```python
from build123d import *

# Parameters (mm, degrees)
MODEL_R             = 1.62599878
MODEL_W             = 8.89
MODEL_H             = 6.096
EXTRUDE_1_DEPTH     = 1
EXTRUDE_2_DEPTH     = 3
SKETCH_1_W          = 8.89
SKETCH_1_H          = 1
EXTRUDE_3_DEPTH     = 0.5
SKETCH_2_W          = 1
SKETCH_2_H          = 5.207
EXTRUDE_4_DEPTH     = 0.5
SKETCH_3_W          = 1
SKETCH_3_H          = 5.207
EXTRUDE_5_DEPTH     = 0.5
SKETCH_4_W          = 7.636
SKETCH_4_H          = 1
CUT_EXTRUDE_1_DEPTH = 0.5


with BuildPart() as part:
    # Model → Extrude 1 (new body)
    with BuildSketch(Plane.XY):
        with BuildLine():
            Line((122.15333456, 67.05953568), (122.15333456, 103.29453306))
            ThreePointArc((122.15333456, 103.29453306), (119.410664993, 110.045001733), (112.66019632, 112.7876713))
            Line((112.66019632, 112.7876713), (83.7431777, 112.7876713))
            ThreePointArc((83.7431777, 112.7876713), (77.016609687, 110.107501601), (74.21120032, 103.43219598))
            Line((74.21120032, 103.43219598), (74.21120032, 67.1865433))
            ThreePointArc((74.21120032, 67.1865433), (76.909728462, 60.481379821), (83.57819454, 57.69339998))
            Line((83.57819454, 57.69339998), (112.78719886, 57.69339998))
            ThreePointArc((112.78719886, 57.69339998), (119.410096357, 60.436638183), (122.15333456, 67.05953568))
        make_face()
        with Locations((115.26482408, 64.6938)):
            Circle(MODEL_R, mode=Mode.SUBTRACT)
        with Locations((81.12722408, 105.9434)):
            Circle(MODEL_R, mode=Mode.SUBTRACT)
        with Locations((115.26482408, 105.9434)):
            Circle(MODEL_R, mode=Mode.SUBTRACT)
        with Locations((81.12722408, 64.6938)):
            Circle(MODEL_R, mode=Mode.SUBTRACT)
        with Locations((105.918, 64.897)):
            Rectangle(MODEL_W, MODEL_H, mode=Mode.SUBTRACT)
        Polygon((102.489, 101.346), (102.489, 106.553), (94.615, 106.553), (93.853, 106.553), (93.853, 101.346), align=None, mode=Mode.SUBTRACT)
        with BuildLine():
            ThreePointArc((77.502, 73.554871436), (78.752768, 70.36450237), (81.893126204, 68.992997458))
            Line((81.893126204, 68.992997458), (114.151129528, 68.992999998))
            ThreePointArc((114.151129528, 68.992999998), (117.34149629, 70.243769219), (118.713, 73.384126091))
            Line((118.713, 73.384126091), (118.713, 95.482375327))
            ThreePointArc((118.713, 95.482375327), (117.462140632, 98.672585067), (114.321868602, 100.044000002))
            Line((114.321868602, 100.044000002), (82.063870472, 100.043997462))
            ThreePointArc((82.063870472, 100.043997462), (78.87350371, 98.793228241), (77.502, 95.652871369))
            Line((77.502, 95.652871369), (77.502, 73.554871436))
        make_face(mode=Mode.SUBTRACT)
    extrude(amount=EXTRUDE_1_DEPTH)

    # Model_3 → Extrude 2 (add)
    with BuildSketch(Plane.XY):
        with BuildLine():
            Line((77.502, 73.554871436), (77.502, 95.652871369))
            ThreePointArc((77.502, 95.652871369), (78.87350371, 98.793228241), (82.063870472, 100.043997462))
            Line((82.063870472, 100.043997462), (114.321868602, 100.044000002))
            ThreePointArc((114.321868602, 100.044000002), (117.462140632, 98.672585067), (118.713, 95.482375327))
            Line((118.713, 95.482375327), (118.713, 73.384126091))
            ThreePointArc((118.713, 73.384126091), (117.34149629, 70.243769219), (114.151129528, 68.992999998))
            Line((114.151129528, 68.992999998), (81.893126204, 68.992997458))
            ThreePointArc((81.893126204, 68.992997458), (78.752768, 70.36450237), (77.502, 73.554871436))
        make_face()
        with BuildLine():
            ThreePointArc((82.042, 98.04399746), (80.272252197, 97.363549602), (79.502, 95.631))
            Line((79.502, 95.631), (79.502, 73.533))
            ThreePointArc((79.502, 73.533), (80.182446941, 71.763250556), (81.91499746, 70.99299746))
            Line((81.91499746, 70.99299746), (114.173, 70.993))
            ThreePointArc((114.173, 70.993), (115.942747803, 71.673447858), (116.713, 73.40599746))
            Line((116.713, 73.40599746), (116.713, 95.50418288))
            ThreePointArc((116.713, 95.50418288), (116.032484318, 97.273814255), (114.29999746, 98.044))
            Line((114.29999746, 98.044), (82.042, 98.04399746))
        make_face(mode=Mode.SUBTRACT)
    extrude(amount=EXTRUDE_2_DEPTH)

    # Sketch 1 → Extrude 3 (add)
    with BuildSketch(Plane.XZ.offset(-67.945)):
        with Locations((105.918, 0.5)):
            Rectangle(SKETCH_1_W, SKETCH_1_H)
    extrude(amount=EXTRUDE_3_DEPTH)

    # Sketch 2 → Extrude 4 (add)
    with BuildSketch(Plane(origin=(93.853, 0, 0), x_dir=(0, 0, -1), z_dir=(1, 0, 0))):
        with Locations((-0.5, 103.9495)):
            Rectangle(SKETCH_2_W, SKETCH_2_H)
    extrude(amount=EXTRUDE_4_DEPTH)

    # Sketch 3 → Extrude 5 (add)
    with BuildSketch(Plane.ZY.offset(-102.489)):
        with Locations((0.5, 103.9495)):
            Rectangle(SKETCH_3_W, SKETCH_3_H)
    extrude(amount=EXTRUDE_5_DEPTH)

    # Sketch 4 → Cut-Extrude 1 (cut)
    with BuildSketch(Plane(origin=(0, 101.346, 0), x_dir=(1, 0, 0), z_dir=(0, 1, 0))):
        with Locations((98.171, -0.5)):
            Rectangle(SKETCH_4_W, SKETCH_4_H)
    extrude(amount=-CUT_EXTRUDE_1_DEPTH, mode=Mode.SUBTRACT)


solid = part.part
```
Here's how the part is built. I have some questions about the finished solid (model axes, mm). A direction names the side the tool comes from. Give positions to 0.01 mm unless a question says otherwise; leave off trailing zeros. Order: outer loops, then holes, each group sorted by start corner. A loop starts at its lowest first (then second) coordinate and runs counter-clockwise, first axis right, second up. Notation, with made-up numbers: M -35.5,6 L 5.5,6 A25 cw 5.5,37 Z; hole C 6,-1.75 d4. An arc over 180 degrees is marked long. Use a Markdown table: item, result. Add a question column.
1. If we mould it in two halves opening along Y, with no side actions, what happens to faces 1 (the cylindrical face through (78.84, 98.76, 1.99)), 2 (the flat face through (93, 103, 1)), 3 (the flat face through (98, 98.044, 1))? For each: +Y half, -Y half, draft (parallel to the pull), parting line (faces both ways), or undercut.
2. On a 3-axis mill with a long thin cutter (end or side, diameter ignored), from which of +Z, -Z, +X, -X, +Y, -Y can I reach the whole of each face in a straight line? I mean faces 4 (the flat face through (98, 68.993, 2)), 5 (the cylindrical face through (116.051, 97.254, 1.479)), 6 (the flat face through (118.713, 85, 2)). Say none if no direction works.
3. Suppose I cut it at C-C (z = 2.2). List the corners of the cut face in (x, y) for me (1 decimal).
4. Suppose I cut it at A-A (x = 109.5). List the corners of the cut face in (y, z) for me (3 decimals).
5. For pin 1 Ø0.5 at (y, z) = (64.5, 0.5) entering from +X; pin 2 Ø0.6 at (x, z) = (99.5, 2.5) entering from -Y; pin 3 Ø1.1 at (y, z) = (104.5, 0.5) entering from -X, each with a flat end and sliding along its axis, tell me the tip position at first contact or that it passes through.
6. I need wall thicknesses on probe 1 along Y at (x, z) = (110.5, 2.5); probe 2 along X at (y, z) = (93, 1.6); probe 3 along Z at (x, y) = (91.5, 67). Which ranges of each line are inside material? Lowest first, please. Write a range as from..to.
7. Suppose I cut it at B-B (y = 75.5). List the corners of the cut face in (x, z) for me.
8. Suppose I cut it at D-D (x = 88). List the corners of the cut face in (y, z) for me, and give its area (3 significant figures).
Results list:
| question | item | result |
|---|---|---|
| 1 | face 1 | +Y half |
| 1 | face 2 | draft |
| 1 | face 3 | undercut |
| 2 | face 4 | +Z, +X, -X, -Y |
| 2 | face 5 | +Z, -Z |
| 2 | face 6 | +Z, +X, +Y, -Y |
| 3 | outline | M 77.5,73.6 A4.5 ccw 81.9,69 L 114.2,69 A4.5 ccw 118.7,73.4 L 118.7,95.5 A4.5 ccw 114.3,100 L 82.1,100 A4.5 ccw 77.5,95.7 Z; hole M 79.5,73.5 A2.5 ccw 81.9,71 L 114.2,71 A2.5 ccw 116.7,73.4 L 116.7,95.5 A2.5 ccw 114.3,98 L 82,98 A2.5 ccw 79.5,95.6 Z |
| 4 | outline | M 57.693,0 L 61.849,0 L 61.849,1 L 57.693,1 Z; M 67.445,0 L 70.993,0 L 70.993,3 L 68.993,3 L 68.993,1 L 67.445,1 Z; M 98.044,0 L 112.788,0 L 112.788,1 L 100.044,1 L 100.044,3 L 98.044,3 Z |
| 5 | pin 1 | stops at x = 121.86 |
| 5 | pin 2 | stops at y = 68.99 |
| 5 | pin 3 | stops at x = 74.23 |
| 6 | probe 1 | y = 68.99..70.99, 98.04..100.04 |
| 6 | probe 2 | x = 77.5..79.5, 116.71..118.71 |
| 6 | probe 3 | z = 0..1 |
| 7 | outline | M 74.21,0 L 79.5,0 L 79.5,3 L 77.5,3 L 77.5,1 L 74.21,1 Z; M 116.71,0 L 122.15,0 L 122.15,1 L 118.71,1 L 118.71,3 L 116.71,3 Z |
| 8 | outline | M 57.69,0 L 70.99,0 L 70.99,3 L 68.99,3 L 68.99,1 L 57.69,1 Z; M 98.04,0 L 112.79,0 L 112.79,1 L 100.04,1 L 100.04,3 L 98.04,3 Z |
| 8 | area | 36.0 mm² |
